Verification items for the finished model (mm, model axes). A direction names the side the tool comes from. Give positions to 0.01 mm unless a question says otherwise; leave off trailing zeros. Write each loop counter-clockwise with the first axis right and the second up, starting at its lowest first coordinate (ties: lowest second). Pieces come first, ordered by that corner, then holes. Notation, with made-up numbers: (88.5, 13) -> (143.5, 13) arc R19 ccw to (143.5, 23) -> close; hole circle Ø6 at (-14, 29.5). An arc over 180 degrees is marked (long way). Use one line per item in the form item = value. Start each with the question number.
(1) Scan lines: L1, parallel to Y at x = 46.5, z = -15.75; L2, parallel to X at y = 10.25, z = -16.25; L3, parallel to X at y = 10, z = -3.25. Record each from-to range of solid material in increasing order.
(2) Section check A-A, the plane x = 44. State how many separate pieces and enclosed holes the cut face has, plus the area to 3 significant figures.
(3) Release check for a two-part mould opening along Z. For faces 3 (the face through (21, 6, -25.959)), 4 (the face through (0, 6, -13)), 5 (the face through (24.311, 9.961, -3.846)), 6 (the face through (26, 7.391, -4)) record: pulls with the +Z half, pulls with the -Z half, needs draft (parallel to the pull), parting line crosses it, or undercut.
(4) Set-up check for faces 1 (the face through (22, 8.839, -4)), 2 (the face through (21, 12.459, -13)): record each of +Z, -Z, +X, -X, +Y, -Y from which the full face is reachable in a straight line by a thin tool's end or side.
(5) Section check B-B, the plane y = 11.25. Record the cut outline in (x, z).
(6) Section check D-D, the plane y = 1. Record the cut outline in (x, z), plus the area to 3 significant figures.
(7) Section check C-C, the plane z = -9.25. Record the cut outline in (x, y), plus the area to 3 significant figures.
(8) Depth check by flat-ended pin: pin 1 Ø0.7 at (x, y) = (45.5, 2) entering from -Z; pin 2 Ø0.7 at (x, y) = (46, 4.5) entering from +Z; pin 3 Ø0.5 at (x, z) = (45.5, -18.5) entering from +Y. Enter the tip coordinate at first touch or a pass-through.
from build123d import *

# Parameters (mm, degrees)
SKETCH1_W          = 42.418
SKETCH1_H          = 25.9588
CASING_DEPTH       = 12.4587
SKETCH2_W          = 0.635
SKETCH2_H          = 0.635
PINS_DEPTH         = 7.1374
PINS_PATTERN_COUNT = 9
PINS_PATTERN_PITCH = 2.54
SKETCH3_R          = 1.2192
LED_DEPTH          = 5.0673
SKETCH4_R          = 1.2192
SCAN_BUTTON_DEPTH  = 3.6195


with BuildPart() as part:
    # Sketch1 → Casing (new body)
    with BuildSketch(Plane(origin=(0, 0, 0), x_dir=(1, 0, 0), z_dir=(0, 1, 0))):
        with Locations((21.209, 12.9794)):
            Rectangle(SKETCH1_W, SKETCH1_H)
    extrude(amount=CASING_DEPTH)

    # Sketch2 → Pins (add)
    with BuildSketch(Plane(origin=(42.418, 0, 0), x_dir=(0, 0, -1), z_dir=(1, 0, 0))):
        with Locations((23.495, 6.858)):
            Rectangle(SKETCH2_W, SKETCH2_H)
        with Locations((23.495, 4.318)):
            Rectangle(SKETCH2_W, SKETCH2_H)
        with Locations((23.495, 1.778)):
            Rectangle(SKETCH2_W, SKETCH2_H)
    pins = extrude(amount=PINS_DEPTH)

    # Pins pattern: Pins ×9
    with Locations(*[(0, 0, i * PINS_PATTERN_PITCH) for i in range(1, PINS_PATTERN_COUNT)]):
        add(pins)

    # Sketch3 → LED (cut)
    with BuildSketch(Plane(origin=(0, 12.4587, 0), x_dir=(1, 0, 0), z_dir=(0, 1, 0))):
        with Locations(Location((25.5016, 3.5814, 0), (0, 0, 270))):
            Circle(SKETCH3_R)
    extrude(amount=-LED_DEPTH, mode=Mode.SUBTRACT)

    # Sketch4 → Scan button (cut)
    with BuildSketch(Plane(origin=(0, 12.4587, 0), x_dir=(1, 0, 0), z_dir=(0, 1, 0))):
        with Locations(Location((21.6789, 4.3434, 0), (0, 0, 270))):
            Circle(SKETCH4_R)
    extrude(amount=-SCAN_BUTTON_DEPTH, mode=Mode.SUBTRACT)


solid = part.part
Completed:
q1.L1 = 1.46 to 2.1, 4 to 4.64, 6.54 to 7.18
q1.L2 = 0 to 42.42
q1.L3 = 0 to 21.14, 22.22 to 24.33, 26.67 to 42.42
q2.separate_pieces = 27
q2.enclosed_holes = 0
q2.area = 10.9 mm²
q3.face_3 = pulls with the -Z half
q3.face_4 = needs draft
q3.face_5 = undercut
q3.face_6 = undercut
q4.face_1 = +Y
q4.face_2 = +Z, -Z, +X, -X, +Y
q5.outline = (0, -25.96) -> (42.42, -25.96) -> (42.42, 0) -> (0, 0) -> close; hole circle Ø2.44 at (21.68, -4.34); hole circle Ø2.44 at (25.5, -3.58)
q6.outline = (0, -25.96) -> (42.42, -25.96) -> (42.42, 0) -> (0, 0) -> close
q6.area = 1,100 mm²
q7.outline = (0, 0) -> (42.42, 0) -> (42.42, 12.46) -> (0, 12.46) -> close
q7.area = 528 mm²
q8.pin_1 = -23.81
q8.pin_2 = -2.86
q8.pin_3 = 7.18
